The model under review builds one solid part; all positions refer to its coordinate system, in mm. A direction names the side the tool comes from. Give positions to 0.01 mm unless a question says otherwise; leave off trailing zeros. Loops run counter-clockwise (first coordinate to the right, second up) from the corner with the lowest first, then second, coordinate; pieces in that order, holes last. Notation, with made-up numbers: (49, 2.5) -> (67, 2.5) arc R30 ccw to (67, 38.5) -> close; hole circle Ø5 at (20.25, 80). An arc over 180 degrees is marked (long way). Write each question's results on one line, items separated by ' | '. Start each with the question number.
Q1. Machinability: for faces 1 (the face through (-15, -8, 3)), 2 (the face through (-2.5, -4.9, 35.5)), 3 (the face through (-11, -4, 18)), which of the approach directions +Z, -Z, +X, -X, +Y, -Y give a long, thin tool a straight path to every point of the face, cutting with its end or side? Answer none if there is none.
Q2. Insertion check: pin 1 Ø4.5 at (x, z) = (-15, 3.5) entering from +Y; pin 2 Ø0.9 at (y, z) = (-2.5, 14.5) entering from -X. Each pin has a flat end and moves straight along its axis. Give the tip position at first contact, or say it passes through.
Q3. We need section C-C (x = -15). Write out the cut boundary in (y, z), plus the area to 3 significant figures.
Q4. We need section A-A (z = 3.5). Write out the cut boundary in (x, y), plus the area to 3 significant figures.
Q5. We need section B-B (y = -4.75). Write out the cut boundary in (x, z).
Q6. Wall thickness on L1, parallel to Z at x = -15, y = -5.4; L2, parallel to Z at x = -15, y = -7.1; L3, parallel to Z at x = -12.5, y = -5.5: over which ranges is each line inside the solid? List them lowest first. Write a range as [from, to].
Q7. Mouldability with a two-part tool opening along X and no side actions: class faces 4 (the face through (-19, -6, 35)), 5 (the face through (-15, -5, 28)), 6 (the face through (-2.5, -9.5, 17.8)) as released by +X, released by -X, zero draft, split by the parting line, or undercut.
Q8. We need section D-D (y = -2.75). Write out the cut boundary in (x, z).
from build123d import *

# Parameters (mm, degrees)
BOX034_W                             = 5.5
BOX034_H                             = 3
BOX034_DEPTH                         = 20
CYLINDER016033_R                     = 1.9
CYLINDER016033_DEPTH                 = 10
CYLINDER016032_R                     = 1.9
CYLINDER016032_DEPTH                 = 10
BOX020_W                             = 14
BOX020_H                             = 9
BOX020_DEPTH                         = 40
BOX019_W                             = 14
BOX019_H                             = 9
BOX019_DEPTH                         = 40
BOX036_W                             = 25.5
BOX036_H                             = 3
BOX036_DEPTH                         = 36
BOX035_W                             = 40
BOX035_H                             = 9
BOX035_DEPTH                         = 36
CHAMFER016016008004017002013003_SIZE = 2
CHAMFER016016008004017002013004_SIZE = 1
CHAMFER016016008004017002013005_SIZE = 1


with BuildPart() as cube034:
    # Box034 → Box034 (new body)
    with BuildSketch(Plane(origin=(-17.75, -7, 8), x_dir=(1, 0, 0), z_dir=(0, 0, 1))):
        with Locations((2.75, 1.5)):
            Rectangle(BOX034_W, BOX034_H)
    extrude(amount=BOX034_DEPTH)


with BuildPart() as cylinder047:
    # Cylinder016033 → Cylinder016033 (new body)
    with BuildSketch(Plane(origin=(-15, 0, 3.5), x_dir=(1, 0, 0), z_dir=(0, 1, 0))):
        Circle(CYLINDER016033_R)
    extrude(amount=CYLINDER016033_DEPTH)


with BuildPart() as fusion018007003008:
    # Cylinder016032 → Cylinder016032 (new body)
    with BuildSketch(Plane(origin=(-15, 0, 32.5), x_dir=(1, 0, 0), z_dir=(0, 1, 0))):
        Circle(CYLINDER016032_R)
    extrude(amount=CYLINDER016032_DEPTH)

    # Fusion018007003008: union Cylinder047
    add(cylinder047.part)


with BuildPart() as fusion018007003008_1:
    # Fusion018007003008 placement: moved
    add(fusion018007003008.part.moved(Location((0, -8, 0))))


with BuildPart() as cube020:
    # Box020 → Box020 (new body)
    with BuildSketch(Plane(origin=(-34, -10, 0), x_dir=(1, 0, 0), z_dir=(0, 0, 1))):
        with Locations((7, 4.5)):
            Rectangle(BOX020_W, BOX020_H)
    extrude(amount=BOX020_DEPTH)


with BuildPart() as cube019:
    # Box019 → Box019 (new body)
    with BuildSketch(Plane(origin=(-2, -10, 0), x_dir=(1, 0, 0), z_dir=(0, 0, 1))):
        with Locations((7, 4.5)):
            Rectangle(BOX019_W, BOX019_H)
    extrude(amount=BOX019_DEPTH)


with BuildPart() as cube036:
    # Box036 → Box036 (new body)
    with BuildSketch(Plane(origin=(-30, -4, 0), x_dir=(1, 0, 0), z_dir=(0, 0, 1))):
        with Locations((12.75, 1.5)):
            Rectangle(BOX036_W, BOX036_H)
    extrude(amount=BOX036_DEPTH)


with BuildPart() as obj1:
    # Box035 → Box035 (new body)
    with BuildSketch(Plane(origin=(-30, -10, 0), x_dir=(1, 0, 0), z_dir=(0, 0, 1))):
        with Locations((20, 4.5)):
            Rectangle(BOX035_W, BOX035_H)
    extrude(amount=BOX035_DEPTH)

    # Cut010011008009003016003: cut Cube036
    add(cube036.part, mode=Mode.SUBTRACT)

    # Cut010011008009003016004: cut Cube019
    add(cube019.part, mode=Mode.SUBTRACT)

    # Cut010011008009003016022: cut Cube020
    add(cube020.part, mode=Mode.SUBTRACT)

    # Chamfer016016008004017002013003
    chamfer016016008004017002013003_edges = [obj1.edges().sort_by_distance(p)[0] for p in [
        (-20, -7, 36),
        (-20, -7, 0),
    ]]
    chamfer(chamfer016016008004017002013003_edges, length=CHAMFER016016008004017002013003_SIZE)

    # Chamfer016016008004017002013004
    chamfer016016008004017002013004_edges = [obj1.edges().sort_by_distance(p)[0] for p in [
        (-2, -5.5, 36),
        (-2, -5.5, 0),
    ]]
    chamfer(chamfer016016008004017002013004_edges, length=CHAMFER016016008004017002013004_SIZE)

    # Cut010011008009003016023: cut Fusion018007003008
    add(fusion018007003008_1.part, mode=Mode.SUBTRACT)

    # Cut010011008009003016024: cut Cube034
    add(cube034.part, mode=Mode.SUBTRACT)

    # Chamfer016016008004017002013005
    chamfer016016008004017002013005_edges = [obj1.edges().sort_by_distance(p)[0] for p in [
        (-10.5, -10, 36),
        (-10.5, -10, 0),
        (-19, -10, 1),
        (-20, -10, 18),
        (-19, -10, 35),
        (-2.5, -10, 35.5),
        (-2, -10, 18),
        (-2.5, -10, 0.5),
    ]]
    chamfer(chamfer016016008004017002013005_edges, length=CHAMFER016016008004017002013005_SIZE)


solid = obj1.part
Output:
1) face 1: +Y | face 2: +Z, +X, +Y, -Y | face 3: +Z, -Z, -X, +Y
2) pin 1: y = -4 | pin 2: x = -4.5
3) outline: (-10, 1) -> (-9, 0) -> (-4, 0) -> (-4, 1.6) -> (-8, 1.6) -> (-8, 5.4) -> (-4, 5.4) -> (-4, 8) -> (-7, 8) -> (-7, 28) -> (-4, 28) -> (-4, 30.6) -> (-8, 30.6) -> (-8, 34.4) -> (-4, 34.4) -> (-4, 36) -> (-9, 36) -> (-10, 35) -> close | area: 125 mm2
4) outline: (-20, -9) -> (-19, -10) -> (-3, -10) -> (-2, -9) -> (-2, -1) -> (-4.5, -1) -> (-4.5, -4) -> (-13.1, -4) -> (-13.1, -8) -> (-16.9, -8) -> (-16.9, -4) -> (-20, -4) -> close | area: 99.3 mm2
5) outline: (-20, 2) -> (-18, 0) -> (-3, 0) -> (-2, 1) -> (-2, 35) -> (-3, 36) -> (-18, 36) -> (-20, 34) -> close; hole (-17.75, 8) -> (-12.25, 8) -> (-12.25, 28) -> (-17.75, 28) -> close; hole circle Ø3.8 at (-15, 3.5); hole circle Ø3.8 at (-15, 32.5)
6) L1: [0, 1.6], [5.4, 8], [28, 30.6], [34.4, 36] | L2: [0, 1.6], [5.4, 30.6], [34.4, 36] | L3: [0, 8], [28, 36]
7) face 4: released by -X | face 5: undercut | face 6: released by +X
8) outline: (-4.5, 0) -> (-3, 0) -> (-2, 1) -> (-2, 35) -> (-3, 36) -> (-4.5, 36) -> close
